from build123d import *

# Parameters (mm, degrees)
F0_R        = 1.5
F1_DEPTH    = 3
F2_R        = 2
F3_R        = 2
F4_T1_DEPTH = 19.5359456942


# Not quite as in the source:
# - a fillet or chamfer that OpenCascade refuses, or shapes differently, is made with other operations: its cross-section is extruded or revolved along the edge and cut away or added


with BuildPart() as f1:
    # F0 (on Front) → F1 (new body)
    with BuildSketch(Plane.XZ):
        Polygon((-14.9506077915, 50.13686046), (-19.9506077915, 50.13686046), (-19.9506077915, 43.13686046), (-18.7006077915, 43.13686046), (-18.7006077915, 10.13686046), (-18.7006077915, -9.86313954), (-17.4506077915, -9.86313954), (-16.2006077915, -9.86313954), (-16.2006077915, 10.13686046), (-16.2006077915, 43.13686046), (-14.9506077915, 43.13686046), align=None)
        with Locations((-17.4506077915, 47.63686046)):
            Circle(F0_R, mode=Mode.SUBTRACT)
    extrude(amount=F1_DEPTH)

    # F2
    f2_edges = [f1.edges().sort_by_distance(p)[0] for p in [
        (-14.950608, -1.5, 50.13686),
    ]]
    fillet(f2_edges, radius=F2_R)

    # F3
    f3_edges = [f1.edges().sort_by_distance(p)[0] for p in [
        (-19.950608, -1.5, 50.13686),
    ]]
    fillet(f3_edges, radius=F3_R)

    # F4: fillet of radius 5 on 2 edges, made by hand

    # F4_s2 → F4_t1 (cut)
    with BuildSketch(Plane.XZ.offset(-8.2679728471)):
        with BuildLine():
            ThreePointArc((-14.9506077915, 46.4440495989), (-15.2735360581, 44.6762826459), (-16.2006077915, 43.13686046))
            Line((-16.2006077915, 43.13686046), (-14.9506077915, 43.13686046))
            Line((-14.9506077915, 43.13686046), (-14.9506077915, 46.4440495989))
        make_face()
        with BuildLine():
            ThreePointArc((-19.9506077915, 46.4440495989), (-19.627679525, 44.6762826459), (-18.7006077915, 43.13686046))
            Line((-18.7006077915, 43.13686046), (-19.9506077915, 43.13686046))
            Line((-19.9506077915, 43.13686046), (-19.9506077915, 46.4440495989))
        make_face()
    extrude(amount=F4_T1_DEPTH, mode=Mode.SUBTRACT)

    # F5 (on face) → F6 (revolve)
    with BuildSketch(Plane(origin=(0, 0, -9.86313954), x_dir=(1, 0, 0), z_dir=(0, 0, -1))):
        with BuildLine():
            Line((-17.4506077915, 3), (-17.4506077915, 6))
            ThreePointArc((-17.4506077915, 6), (-21.9506077915, 1.5), (-17.4506077915, -3))
            Line((-17.4506077915, -3), (-17.4506077915, 0))
            Line((-17.4506077915, 0), (-18.7006077915, 0))
            Line((-18.7006077915, 0), (-18.7006077915, 3))
            Line((-18.7006077915, 3), (-17.4506077915, 3))
        make_face()
    revolve(axis=Axis((-17.4506077915, -1.5, -9.86313954), (0, 1, 0)))


solid = f1.part
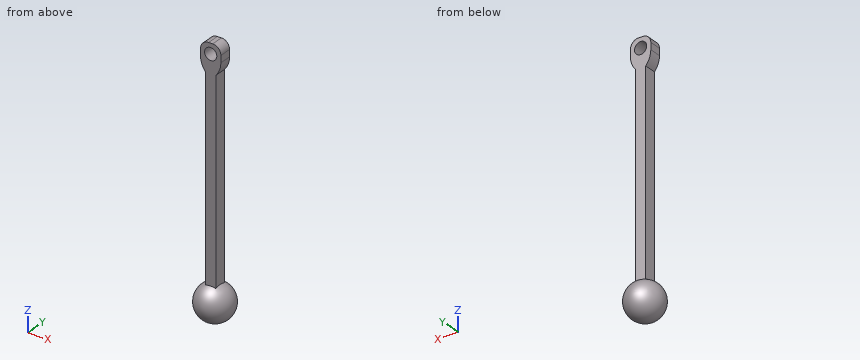
Design review of the part built by this model. Coordinates are the model's own, in mm. Round coordinates to 2 decimals unless told otherwise and drop trailing zeros. Loops run counter-clockwise (first coordinate to the right, second up) from the corner with the lowest first, then second, coordinate; pieces in that order, holes last. Notation, with made-up numbers: (-1, 63) -> (51, 63) arc R17 ccw to (51, 73) -> close; hole circle Ø1 at (45.25, -9.5). An arc over 180 degrees is marked (long way). Use one line per item in the form item = value. Start each with the question number.
Q1. We need section A-A on z = -8. Give the boundary of the cut face in (x, y).
Q2. We need section B-B on x = -14.25. Give the boundary of the cut face in (y, z), then the cut area to 3 significant figures.
Q3. For pin 1 Ø1.5 at (y, z) = (0, 24) entering from +X; pin 2 Ø4 at (x, z) = (-15.5, 17.5) entering from -Y; pin 3 Ø4 at (y, z) = (-2, 6.5) entering from -X, all flat-tipped, find the tip position at first contact; note any pin that passes through.
Q4. Wall thickness on line 1 along Y through (x, z) = (-17.25, 45.5); line 2 along Z through (x, y) = (-18.75, -2.5); line 3 along X through (y, z) = (-1, 29.5): over which ranges is each line inside the solid? List them lowest first. Write a range as [from, to].
Calculated:
q1.outline = circle Ø8.19 at (-17.45, -1.5)
q2.outline = circle Ø6.33 at (-1.5, -9.86)
q2.area = 31.4 mm²
q3.pin_1 = -16.2
q3.pin_2 = -3
q3.pin_3 = -18.7
q4.line_1 = [-3, 0]
q4.line_2 = [-14.05, -5.67], [43.19, 46.89], [48.39, 49.97]
q4.line_3 = [-18.7, -16.2]
